The model under review builds one solid part; all positions refer to its coordinate system, in mm. Round coordinates to 2 decimals unless told otherwise and drop trailing zeros. Order: outer loops, then holes, each group sorted by start corner. A loop starts at its lowest first (then second) coordinate and runs counter-clockwise, first axis right, second up.
1) Clearance check with flat-ended pins moving along their axes: P1, Ø1.5, axis at x = -24.5, y = 17.5, coming from the -Z side; P2, Ø8, axis at x = -54.5, y = 8, coming from the -Z side; P3, Ø5, axis at x = 6.5, y = 16.5, coming from the +Z side. State where each tip first meets the part, or that it passes through.
2) Consider section C-C (y = 8.5). Give the boundary of the cut face in (x, z), then the cut area to 3 significant figures.
3) To check wall thickness, follow L1, parallel to X at y = 2.75, z = 44; L2, parallel to Z at x = -8.5, y = 18.5; L3, parallel to Y at x = 78, z = 93.5. State the ranges of each line that lie inside material, in increasing order.
Autodesk Inventor part; units mm, degrees
ref_plane "YZ Plane" through (0, 0, 0) normal (1, 0, 0) x (0, 1, 0)
ref_plane "XZ Plane" through (0, 0, 0) normal (0, 1, 0) x (-1, 0, 0)
ref_plane "XY Plane" through (0, 0, 0) normal (0, 0, 1) x (1, 0, 0)
sketch "Sketch1" plane through (0, 0, 0) normal (0, 1, 0) x (-1, 0, 0)
  line L0 (87.95, 138.75) -> (-87.95, 138.75)
  line L1 (-87.95, 138.75) -> (-87.95, -138.75)
  line L2 (-87.95, -138.75) -> (87.95, -138.75)
  line L3 (87.95, -138.75) -> (87.95, 138.75)
  line L4 (87.95, 138.75) -> (-87.95, -138.75) construction
  line L5 (-87.95, 138.75) -> (87.95, -138.75) construction
  point P0 (0, 0)
  dimension "d0" = 175.9
  dimension "d1" = 277.5
extrude "Extrusion1" add sketch "Sketch1" along normal blind 20
chamfer "Chamfer3" distance 20 angle 45 3 edges at (0, 20, 138.75) (0, 20, -138.75) (87.95, 20, 0)
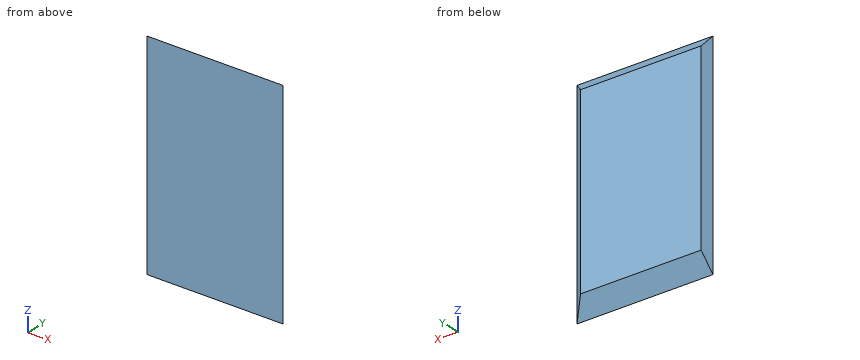
Answer below:
1. P1: stops at z = -122
1. P2: stops at z = -134.75
1. P3: stops at z = 124.75
2. outline: (-87.95, -130.25) - (79.45, -130.25) - (79.45, 130.25) - (-87.95, 130.25) - close
2. area: 43,600 mm2
3. L1: x = -87.95 to 85.2
3. L2: z = -120.25 to 120.25
3. L3: y = 0 to 9.95
